```python
from build123d import *

# Parameters (mm, degrees)
SKETCH_1_R               = 50
EXTRUDE_1_DEPTH          = 200
CUT_EXTRUDE_1_DEPTH      = 200
CUT_EXTRUDE_1_DEPTH_BACK = 200
CUT_EXTRUDE_4_DEPTH      = 200
CUT_EXTRUDE_4_DEPTH_BACK = 200
CUT_EXTRUDE_5_DEPTH      = 200
CUT_EXTRUDE_5_DEPTH_BACK = 200
SKETCH_5_R               = 15


with BuildPart() as part:
    # Sketch 1 → Extrude 1 (new body)
    with BuildSketch(Plane(origin=(0, 0, 0), x_dir=(1, 0, 0), z_dir=(0, 1, 0))):
        with Locations(Location((0, 0, 0), (0, 0, 270))):
            Circle(SKETCH_1_R)
    extrude(amount=EXTRUDE_1_DEPTH)

    # Sketch 2 → Cut-Extrude 1 (cut, two sides: drawn at the far end of the back side and taken through both)
    with BuildSketch(Plane(origin=(0, 0, 0), x_dir=(0, 0, -1), z_dir=(1, 0, 0)).offset(-CUT_EXTRUDE_1_DEPTH_BACK)):
        Polygon((-70, 250), (70, 250), (70, 100), (20, 100), (20, 240), (-20, 240), (-20, 100), (-70, 100), align=None)
    extrude(amount=CUT_EXTRUDE_1_DEPTH + CUT_EXTRUDE_1_DEPTH_BACK, mode=Mode.SUBTRACT)

    # Sketch 3 → Cut-Extrude 4 (cut, two sides: drawn at the far end of the back side and taken through both)
    with BuildSketch(Plane.XY.offset(20).offset(-CUT_EXTRUDE_4_DEPTH_BACK)):
        with BuildLine():
            Line((50, 150), (108.18036677, 150))
            Line((108.18036677, 150), (108.18036677, 270))
            Line((108.18036677, 270), (-86.328849113, 270))
            Line((-86.328849113, 270), (-86.328849113, 150))
            Line((-86.328849113, 150), (-50, 150))
            ThreePointArc((-50, 150), (0, 200), (50, 150))
        make_face()
    extrude(amount=CUT_EXTRUDE_4_DEPTH + CUT_EXTRUDE_4_DEPTH_BACK, mode=Mode.SUBTRACT)

    # Sketch 5 → Cut-Extrude 5 (cut, two sides: drawn at the far end of the back side and taken through both)
    with BuildSketch(Plane.XY.offset(20).offset(-CUT_EXTRUDE_5_DEPTH_BACK)):
        with Locations(Location((0, 150, 0), (0, 0, 180))):
            Circle(SKETCH_5_R)
    extrude(amount=CUT_EXTRUDE_5_DEPTH + CUT_EXTRUDE_5_DEPTH_BACK, mode=Mode.SUBTRACT)


solid = part.part
```
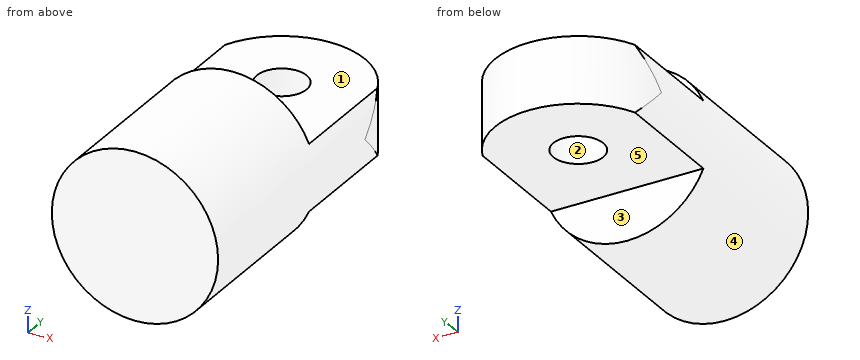
Can you work these out from the model? Positions are in its coordinate system, mm. Face numbers are marked on the shaded views. A direction names the side the tool comes from. Give positions to 0.01 mm unless a question says otherwise; leave off trailing zeros. Order: outer loops, then holes, each group sorted by start corner. A loop starts at its lowest first (then second) coordinate and runs counter-clockwise, first axis right, second up. Notation, with made-up numbers: M -30,-11.5 L 4,-11.5 A33 cw 4,27.5 Z; hole C -33,-33 d10. An arc over 180 degrees is marked long. Write item = value, one per line. Start each with the question number.
Q1. Suppose I cut it at C-C (y = 145). Write out the boundary of the cut face in (x, z).
Q2. Will these pins go through, and if not, where does the flat tip stop? pin 1 Ø3 at (y, z) = (78.5, 30.5) entering from +X; pin 2 Ø8 at (x, y) = (-35.5, 43) entering from +Z; pin 3 Ø4 at (x, y) = (23.5, 143) entering from -Z.
Q3. We'd pull the mould along Y, two halves only. Please class the marked faces 1, 2 and 3: pulls with the +Y half, pulls with the -Y half, needs draft (parallel to the pull), parting line crosses it, or undercut.
Q4. Suppose I cut it at D-D (x = 43). Write out the boundary of the cut face in (y, z).
Q5. I need wall thicknesses on probe 1 along Z at (x, y) = (-41.5, 109); probe 2 along Y at (x, z) = (-26.5, 26.5); probe 3 along Z at (x, y) = (-1, 22). Which ranges of each line are inside material? Lowest first, please. Write a range as [from, to].
Q6. Suppose I cut it at B-B (z = 0). Write out the boundary of the cut face in (x, y).
Q7. For the marked faces 4 and 5, which set-ups out of +Z, -Z, +X, -X, +Y, -Y let a thin tool reach every point of the face, with its end or its side?
Q8. Suppose I cut it at A-A (x = 0). Write out the boundary of the cut face in (y, z), plus the area to 3 significant figures.
Check result:
q1.outline = M -45.83,-20 L -14.14,-20 L -14.14,20 L -45.83,20 A50 ccw Z; M 14.14,-20 L 45.83,-20 A50 ccw 45.83,20 L 14.14,20 Z
q2.pin_1 = 40.73
q2.pin_2 = 38.83
q2.pin_3 = -20
q3.face_1 = needs draft
q3.face_2 = undercut
q3.face_3 = pulls with the +Y half
q4.outline = M 0,-25.51 L 100,-25.51 L 100,-20 L 175.51,-20 L 175.51,20 L 100,20 L 100,25.51 L 0,25.51 Z
q5.probe_1 = [-20, 20]
q5.probe_2 = [0, 100]
q5.probe_3 = [-49.99, 49.99]
q6.outline = M -50,0 L 50,0 L 50,150 A50 ccw -50,150 Z; hole C 0,150 d30
q7.face_4 = +Y, -Y
q7.face_5 = -Z, +X, -X, +Y
q8.outline = M 0,-50 L 100,-50 L 100,-20 L 135,-20 L 135,20 L 100,20 L 100,50 L 0,50 Z; M 165,-20 L 200,-20 L 200,20 L 165,20 Z
q8.area = 12,800 mm2
